from build123d import *

# Parameters (mm, degrees)
SKETCH2_R          = 17.5
CUT_EXTRUDE1_DEPTH = 108.121426428
SKETCH3_W          = 10
SKETCH3_H          = 6.6
CUT_EXTRUDE2_DEPTH = 108.121426428
SKETCH4_R          = 4
CUT_EXTRUDE3_DEPTH = 10
SKETCH6_R          = 81.550028755
CUT_EXTRUDE6_DEPTH = 60


with BuildPart() as part:
    # Sketch1 → Revolve1 (revolve)
    with BuildSketch(Plane.XY, mode=Mode.PRIVATE) as revolve1_sk:
        with BuildLine():
            Line((-55, 0), (0, 0))
            Line((0, 0), (0, 65))
            Line((0, 65), (-15, 65))
            ThreePointArc((-15, 65), (-18.535533906, 63.535533906), (-20, 60))
            Line((-20, 60), (-20, 38))
            ThreePointArc((-20, 38), (-22.343145751, 32.343145751), (-28, 30))
            Line((-28, 30), (-52, 30))
            ThreePointArc((-52, 30), (-54.121320344, 29.121320344), (-55, 27))
            Line((-55, 27), (-55, 0))
        make_face()
    revolve(revolve1_sk.sketch.rotate(Axis((-55, 0, 0), (1, 0, 0)), 90), axis=Axis((-55, 0, 0), (1, 0, 0)))

    # Sketch2 → Cut-Extrude1 (cut, through all)
    with BuildSketch(Plane.ZY.offset(55)):
        Circle(SKETCH2_R)
    extrude(amount=-CUT_EXTRUDE1_DEPTH, mode=Mode.SUBTRACT)

    # Sketch3 → Cut-Extrude2 (cut, through all)
    with BuildSketch(Plane(origin=(0, 0, 0), x_dir=(0, 0, -1), z_dir=(1, 0, 0))):
        with Locations((0, 17.5)):
            Rectangle(SKETCH3_W, SKETCH3_H)
    extrude(amount=-CUT_EXTRUDE2_DEPTH, mode=Mode.SUBTRACT)

    # Sketch4 → Cut-Extrude3 (cut)
    with BuildSketch(Plane(origin=(0, -30, 0), x_dir=(-1, 0, 0), z_dir=(0, -1, 0))):
        with Locations(Location((40.229772479, 0, 0), (0, 0, 90))):
            Circle(SKETCH4_R)
    extrude(amount=-CUT_EXTRUDE3_DEPTH, mode=Mode.SUBTRACT)

    # Cut-Extrude5 cone 1 section (through the dimple's axis) → Cut-Extrude5 (revolve, cut)
    with BuildSketch(Plane(origin=(0, 47.5, 0), x_dir=(0, 0, -1), z_dir=(0, 1, 0))):
        Polygon((0, 0), (7, 0), (0, 93.336682434), align=None)
    revolve(axis=Axis((0, 47.5, 0), (-1, 0, 0)), mode=Mode.SUBTRACT)

    # Cut-Extrude5 cone 2 section (through the dimple's axis) → Cut-Extrude5 cone 2 (revolve, cut)
    with BuildSketch(Plane(origin=(0, -23.75, -41.13620668), x_dir=(0, 0, -1), z_dir=(0, 1, 0))):
        Polygon((0, 0), (7, 0), (0, 93.336682434), align=None)
    revolve(axis=Axis((0, -23.75, -41.13620668), (-1, 0, 0)), mode=Mode.SUBTRACT)

    # Cut-Extrude5 cone 3 section (through the dimple's axis) → Cut-Extrude5 cone 3 (revolve, cut)
    with BuildSketch(Plane(origin=(0, -23.75, 41.13620668), x_dir=(0, 0, -1), z_dir=(0, 1, 0))):
        Polygon((0, 0), (7, 0), (0, 93.336682434), align=None)
    revolve(axis=Axis((0, -23.75, 41.13620668), (-1, 0, 0)), mode=Mode.SUBTRACT)

    # Mirror1: part across plane


with BuildPart() as part_1:
    add(part.part)
    add(part.part.mirror(Plane.ZY))

    # Sketch6 → Cut-Extrude6 (cut)
    with BuildSketch(Plane(origin=(0, 0, 0), x_dir=(0, 0, -1), z_dir=(1, 0, 0))):
        Circle(SKETCH6_R)
    extrude(amount=-CUT_EXTRUDE6_DEPTH, mode=Mode.SUBTRACT)


solid = part_1.part
Check sheet for the modelled part. Datum: model origin and axes. Units: mm. A direction names the side the tool comes from. Coordinates: 2 decimals unless noted, no trailing zeros. Loops run counter-clockwise (first coordinate to the right, second up) from the corner with the lowest first, then second, coordinate; pieces in that order, holes last. Notation, with made-up numbers: (-33.5, -37.75) -> (19.5, -37.75) arc R19 cw to (19.5, -33.75) -> close; hole circle Ø1 at (75, -34.5). An arc over 180 degrees is marked (long way). Write item = value, one per line. Start each with the question number.
1. Draft check along X on faces 5 (the flat face through (27, 20.8, 0)), 6 (the flat face through (40, -20, 0)), 7 (the conical face through (10.14, 53.59, 1.35)). Enter one of: released by +X, released by -X, zero draft, split by the parting line, or undercut.
2. Material ranges on line 1 (X direction, y = -27.25, z = 0); line 2 (X direction, y = -56, z = 0.5); line 3 (Y direction, x = 48, z = 1), recorded low to high.
3. Section check B-B on z = 0. Record the cut outline in (x, y).
4. Section check A-A on y = 0. Record the cut outline in (x, z), then the cut area to 3 significant figures.
5. Section check D-D on x = 10.5. Record the cut outline in (y, z), then the cut area to 3 significant figures.
6. Section check C-C on x = 46.5. Record the cut outline in (y, z), then the cut area to 3 significant figures.
7. Tool access check on faces 1 (the flat face through (0, -14, -14)), 2 (the cylindrical face through (44.135, -25.071, 0.867)), 3 (the flat face through (20, -1, 39)), 4 (the flat face through (27, 19, -5)). Record the directions out of +Z, -Z, +X, -X, +Y, -Y that give a thin tool (end or side, any length) a straight path to the whole face; none if there is none.
8. Depth check by flat-ended pin: P1, Ø6, axis at y = -47.5, z = 35.5, coming from the +X side; P2, Ø3, axis at x = 23.5, y = 19.5, coming from the +Z side; P3, Ø6, axis at x = 6.5, z = -43.5, coming from the -Y side. Enter the tip coordinate at first touch or a pass-through.
Responses:
q1.face_5 = zero draft
q1.face_6 = undercut
q1.face_7 = released by -X
q2.line_1 = 0 to 36.23, 44.23 to 54.99
q2.line_2 = 0 to 20
q2.line_3 = -29.98 to -17.47, 20.8 to 29.98
q3.outline = (0, -65) -> (15, -65) arc R5 ccw to (20, -60) -> (20, -38) arc R8 cw to (28, -30) -> (36.23, -30) -> (36.23, -20) -> (44.23, -20) -> (44.23, -30) -> (52, -30) arc R3 ccw to (55, -27) -> (55, -17.5) -> (0, -17.5) -> close; (0, 20.8) -> (55, 20.8) -> (55, 27) arc R3 ccw to (52, 30) -> (28, 30) arc R8 cw to (20, 38) -> (20, 42) -> (0, 40.5) -> close; (0, 54.5) -> (20, 53) -> (20, 60) arc R5 ccw to (15, 65) -> (0, 65) -> close
q4.outline = (0, -65) -> (15, -65) arc R5 ccw to (20, -60) -> (20, -38) arc R8 cw to (28, -30) -> (52, -30) arc R3 ccw to (55, -27) -> (55, -17.5) -> (0, -17.5) -> close; (0, 17.5) -> (55, 17.5) -> (55, 27) arc R3 ccw to (52, 30) -> (28, 30) arc R8 cw to (20, 38) -> (20, 60) arc R5 ccw to (15, 65) -> (0, 65) -> close
q4.area = 2,790 mm2
q5.outline = circle Ø130 at (0, 0); hole circle Ø12.43 at (-23.75, -41.14); hole circle Ø12.43 at (-23.75, 41.14); hole (16.77, -5) -> (20.8, -5) -> (20.8, 5) -> (16.77, 5) arc R17.5 ccw (long way) to start; hole circle Ø12.43 at (47.5, 0)
q5.area = 11,900 mm2
q6.outline = circle Ø60 at (0, 0); hole (16.77, -5) -> (20.8, -5) -> (20.8, 5) -> (16.77, 5) arc R17.5 ccw (long way) to start
q6.area = 1,830 mm2
q7.face_1 = +Z, -Z, -X, +Y, -Y
q7.face_2 = -Y
q7.face_3 = +X
q7.face_4 = +X, -X
q8.P1 = 20
q8.P2 = 26.53
q8.P3 = -50.84
